```python
from build123d import *

# Parameters (mm, degrees)
SKETCH_1_R                   = 75
EXTRUDE_1_DEPTH              = 10
SKETCH_2_R                   = 35
SKETCH_2_R_2                 = 25
EXTRUDE_1_2_DEPTH            = 250
HOLE_WIZARD_1_D              = 25
HOLE_WIZARD_M5_1_D           = 4.2
HOLE_WIZARD_M5_1_DEPTH       = 22.4
HOLE_WIZARD_M5_1_CSINK_D     = 5.05
HOLE_WIZARD_M5_1_CSINK_ANGLE = 90
HOLE_WIZARD_M5_1_TIP         = 1.2618073
FILLET_1_R                   = 5


with BuildPart() as part:
    # 草图1 → Extrude 1 (new body)
    with BuildSketch(Plane(origin=(0, 0, 0), x_dir=(1, 0, 0), z_dir=(0, 1, 0))):
        with Locations(Location((0, 0, 0), (0, 0, 270))):
            Circle(SKETCH_1_R)
    extrude(amount=EXTRUDE_1_DEPTH)

    # 草图2 → Extrude 1 2 (add)
    with BuildSketch(Plane(origin=(0, 10, 0), x_dir=(1, 0, 0), z_dir=(0, 1, 0))):
        Circle(SKETCH_2_R)
        Circle(SKETCH_2_R_2, mode=Mode.SUBTRACT)
    extrude(amount=EXTRUDE_1_2_DEPTH)

    # 孔1 (through all)
    with Locations(Plane(origin=(0, 10, 0), x_dir=(1, 0, 0), z_dir=(0, 1, 0))):
        with Locations((0, 57.5), (57.5, 0), (0, -57.5), (-57.5, 0)):
            Hole(HOLE_WIZARD_1_D / 2)

    # M5 螺纹孔1
    with Locations(Plane(origin=(0, 260, 0), x_dir=(1, 0, 0), z_dir=(0, 1, 0))):
        with Locations((0, -30), (-30, 0), (0, 30), (30, 0)):
            CounterSinkHole(HOLE_WIZARD_M5_1_D / 2, HOLE_WIZARD_M5_1_CSINK_D / 2, depth=HOLE_WIZARD_M5_1_DEPTH, counter_sink_angle=HOLE_WIZARD_M5_1_CSINK_ANGLE)
            with Locations((0, 0, -(HOLE_WIZARD_M5_1_DEPTH + HOLE_WIZARD_M5_1_TIP / 2))):  # 118° drill point
                Cone(0, HOLE_WIZARD_M5_1_D / 2, HOLE_WIZARD_M5_1_TIP, mode=Mode.SUBTRACT)

    # 圆角1
    fillet_1_edges = [part.edges().sort_by_distance(p)[0] for p in [
        (-35, 10, 0),
    ]]
    fillet(fillet_1_edges, radius=FILLET_1_R)


solid = part.part
```
Build history of the part. All positions in model axes, mm. A direction names the side the tool comes from. Give positions to 0.01 mm unless a question says otherwise; leave off trailing zeros. Loops run counter-clockwise (first coordinate to the right, second up) from the corner with the lowest first, then second, coordinate; pieces in that order, holes last.
Item 1: Slice it at B-B, the plane x = 57.5. List the corners of the cut face in (y, z), and give its area (3 significant figures).
Answers follow:
outline: (0, -48.15) - (10, -48.15) - (10, -12.5) - (0, -12.5) - close; (0, 12.5) - (10, 12.5) - (10, 48.15) - (0, 48.15) - close
area: 713 mm2
Item 2: Pull direction X, two halves, no side cores. Call faces 3 (the face through (-32, 10, 32)), 4 (the face through (69.988, 4.93, -0.55)), 5 (the face through (1.627, 4.93, 45.106)), 6 (the face through (-45.636, 4.93, -59.517)): released by +X, released by -X, zero draft, split by the parting line, or undercut.
Answers follow:
face 3: zero draft
face 4: undercut
face 5: undercut
face 6: split by the parting line
Item 3: Which spindle directions (+Z, -Z, +X, -X, +Y, -Y) get a long thin tool onto all of the face, cutting with end or side? Do faces 1 (the face through (23, 260, -11)), 2 (the face through (23.846, 133.25, -7.509)). Say none if no direction does.
Answers follow:
face 1: +Z, -Z, +X, -X, +Y
face 2: +Y
Item 4: Slice it at A-A, the plane z = -52.5. List the corners of the cut face in (x, y), and give its area (3 significant figures).
Answers follow:
outline: (-53.56, 0) - (-11.46, 0) - (-11.46, 10) - (-53.56, 10) - close; (11.46, 0) - (53.56, 0) - (53.56, 10) - (11.46, 10) - close
area: 842 mm2
Item 5: Flat gauge pins, fed straight in: pin 1 (12 mm diameter, centred on x = 26.5, z = -40, fed in from +Y); pin 2 (1 mm diameter, centred on x = -19, y = 64.5, fed in from +Z); pin 3 (8 mm diameter, centred on y = 211.5, z = 29.5, fed in from +X). Where does each tip first touch, or does it go through?
Answers follow:
pin 1: stops at y = 10
pin 2: stops at z = 29.71
pin 3: stops at x = 23.97
Item 6: Drill centre lines: line 1 (Z direction, x = 0, y = 112); line 2 (Y direction, x = 18, z = 66). Where is each one in solid material? Low to high.
Answers follow:
line 1: z = -35 to -25, 25 to 35
line 2: y = 0 to 10
Item 7: Slice it at C-C, the plane y = 66. List the corners of the cut face in (x, z), and give its area (3 significant figures).
Answers follow:
outline: circle Ø70 at (0, 0); hole circle Ø50 at (0, 0)
area: 1,880 mm2
